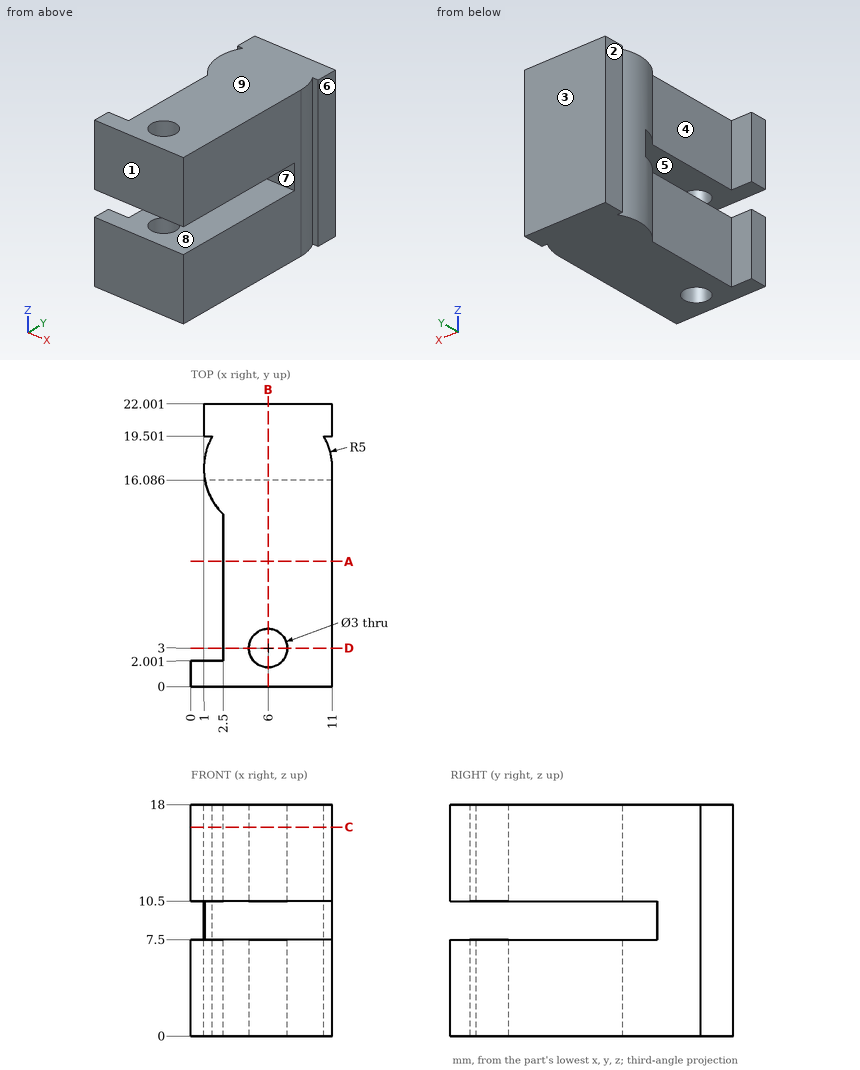
Design review of the part shown in the three views and the two pictorial views. Dimensions are in mm from the part's minimum x, y and z. A direction names the side the tool comes from. Give positions to 0.01 mm unless a question says otherwise; leave off trailing zeros. Write each loop counter-clockwise with the first axis right and the second up, starting at its lowest first coordinate (ties: lowest second). Pieces come first, ordered by that corner, then holes.
(1) Mouldability with a two-part tool opening along Z and no side actions: class the marked faces 6, 7, 8 and 9 as +Z half, -Z half, draft (parallel to the pull), parting line (faces both ways), or undercut.
Checked values:
face 6: draft
face 7: undercut
face 8: undercut
face 9: +Z half
(2) Clearance check with flat-ended pins moving along their axes: pin 1 Ø4 at (y, z) = (6, 14.5) entering from -X; pin 2 Ø10 at (y, z) = (12, 4.5) entering from -X. State where each tip first meets the part, or that it passes through.
Checked values:
pin 1: stops at x = 2.5
pin 2: stops at x = 1
(3) Tool access review of the marked faces 1, 2, 3, 4 and 5: name each direction out of +Z, -Z, +X, -X, +Y, -Y from which nothing blocks a thin tool from reaching the whole face with its end or side.
Checked values:
face 1: +Z, -Z, +X, -X, -Y
face 2: +Z, -Z, -X, +Y
face 3: +Z, -Z, +X, -X, +Y
face 4: +Z, -Z, -X
face 5: +X, -X, -Y
(4) Add section A-A (y = 9.75). Give the boundary of the cut face in (x, z).
Checked values:
outline: (2.5, 0) - (11, 0) - (11, 7.5) - (2.5, 7.5) - close; (2.5, 10.5) - (11, 10.5) - (11, 18) - (2.5, 18) - close
(5) Add section C-C (z = 16.25). Give the boundary of the cut face in (x, y), and give its area (3 significant figures).
Checked values:
outline: (0, 0) - (11, 0) - (11, 17) arc R5 ccw to (10.33, 19.5) - (11, 19.5) - (11, 22) - (1, 22) - (1, 19.5) - (1.67, 19.5) arc R5 ccw to (2.5, 13.43) - (2.5, 2) - (0, 2) - close; hole circle Ø3 at (6, 3)
area: 195 mm2
(6) Wall thickness on line 1 along X through (y, z) = (3, 3.75); line 2 along Z through (x, y) = (9, 13.5); line 3 along Y through (x, z) = (6, 3): over which ranges is each line inside the solid? List them lowest first.
Checked values:
line 1: x = 2.5 to 4.5, 7.5 to 11
line 2: z = 0 to 7.5, 10.5 to 18
line 3: y = 0 to 1.5, 4.5 to 22
(7) Add section B-B (x = 6). Give the boundary of the cut face in (y, z) (1 decimal), and give its area (3 significant figures).
Checked values:
outline: (0, 0) - (1.5, 0) - (1.5, 7.5) - (0, 7.5) - close; (0, 10.5) - (1.5, 10.5) - (1.5, 18) - (0, 18) - close; (4.5, 0) - (22, 0) - (22, 18) - (4.5, 18) - (4.5, 10.5) - (16.1, 10.5) - (16.1, 7.5) - (4.5, 7.5) - close
area: 303 mm2
(8) Add section D-D (y = 3). Give the boundary of the cut face in (x, z).
Checked values:
outline: (2.5, 0) - (4.5, 0) - (4.5, 7.5) - (2.5, 7.5) - close; (2.5, 10.5) - (4.5, 10.5) - (4.5, 18) - (2.5, 18) - close; (7.5, 0) - (11, 0) - (11, 7.5) - (7.5, 7.5) - close; (7.5, 10.5) - (11, 10.5) - (11, 18) - (7.5, 18) - close
